Can you work these out from the model? Positions are in its coordinate system, mm. A direction names the side the tool comes from. Coordinates: 2 decimals unless noted, no trailing zeros. Order: outer loops, then holes, each group sorted by start corner. A loop starts at its lowest first (then second) coordinate and runs counter-clockwise, first axis right, second up. Notation, with made-up numbers: (33.25, 73) -> (86.25, 73) arc R20 cw to (86.25, 106) -> close; hole circle Ø9 at (22.25, 46). An arc over 180 degrees is marked (long way). Use a Markdown table: item, result. Add a question column.
1. Suppose I cut it at C-C, the plane z = 7. List the corners of the cut face in (x, y) for me.
2. Suppose I cut it at B-B, the plane y = 62.5. List the corners of the cut face in (x, z) for me, then the cut area to 3 significant figures.
3. If I drill on line 1 along Y through (x, z) = (0, -8); line 2 along X through (y, z) = (-31.25, -0.2); line 3 along Z through (x, y) = (33, 12.5), over which ranges is the centre line in solid material (lowest first)? Write a range as from..to.
4. For faces 4 (the flat face through (-17, -46, 1)), 5 (the flat face through (-45, -16, -9)), 6 (the cylindrical face through (-11.923, 53.692, -6.535)), which set-ups out of +Z, -Z, +X, -X, +Y, -Y let a thin tool reach every point of the face, with its end or its side?
5. We'd pull the mould along X, two halves only. Please class faces 1 (the cylindrical face through (-28, -21, 7)), 2 (the flat face through (-37, -41, -4)), 3 (the conical face through (-9, 40, 8)): pulls with the +X half, pulls with the -X half, needs draft (parallel to the pull), parting line crosses it, or undercut.
6. For pin 1 Ø11.5 at (x, y) = (54.13, -31.25) entering from +Z; pin 2 Ø8 at (x, z) = (-9, -7) entering from -Y; pin 3 Ø6 at (x, z) = (42, -2) entering from -Y; pin 4 Ø6 at (x, y) = (-20, 38) entering from +Z, each with a flat end and sliding along its axis, tell me the tip position at first contact or that it passes through.
Autodesk Inventor part; units mm, degrees
ref_plane "YZ Plane" through (0, 0, 0) normal (1, 0, 0) x (0, 1, 0)
ref_plane "XZ Plane" through (0, 0, 0) normal (0, 1, 0) x (-1, 0, 0)
ref_plane "XY Plane" through (0, 0, 0) normal (0, 0, 1) x (1, 0, 0)
sketch "Sketch1" plane through (-195.9052, -159.4976, -9) normal (0, 0, 1) x (1, 0, 0)
  circle A0 centre (195.9052, 159.4976) radius 70
  dimension "d29" = 140
extrude "ExtrusionBlind1" add sketch "Sketch1" along normal blind 18
sketch "Sketch2" plane through (-195.9052, -159.4976, -9) normal (0, 0, 1) x (1, 0, 0)
  circle A0 centre (195.9052, 159.4976) radius 55
  circle A1 centre (195.9052, 159.4976) radius 83.1126
  circle A2 centre (195.9052, 159.4976) radius 70
  dimension "d30" = 166.2252
  dimension "d31" = 110
extrude "ExtrusionBlind2" cut sketch "Sketch2" along normal blind 5 contours A1 | A2
sketch "Sketch3" plane through (-195.9052, -159.4976, -9) normal (0, 0, 1) x (1, 0, 0)
  circle A0 centre (195.9052, 159.4976) radius 30
  circle A1 centre (195.9052, 159.4976) radius 55
  dimension "d32" = 60
extrude "ExtrusionThru1" cut sketch "Sketch3" along normal through all contours A0
sketch "Sketch4" plane through (-195.9052, -159.4976, -9) normal (0, 0, 1) x (1, 0, 0)
  circle A0 centre (195.9052, 159.4976) radius 37.5
  circle A1 centre (195.9052, 159.4976) radius 55
  dimension "d33" = 75
extrude "ExtrusionBlind3" cut sketch "Sketch4" along normal blind 11 contours A0
sketch "Sketch5" plane through (-195.9052, -159.4976, -9) normal (0, 0, 1) x (1, 0, 0)
  circle A0 centre (195.9052, 159.4976) radius 47.5
  circle A1 centre (195.9052, 159.4976) radius 55
  dimension "d34" = 95
extrude "ExtrusionBlind4" cut sketch "Sketch5" along normal blind 3 contours A0
sketch "Sketch6" plane through (0, 0, -4) normal (0, 0, -1) x (-1, 0, 0)
  point P0 (0, -62.5)
hole "Hole1" at (0, -62.5, -4) direction (0, 0, 1) diameter 9 end through all
pattern_circular "PolarArray1" count 6 over 360 about axis through (0, 0, -9) along (0, 0, -1) of "Hole1"
sketch "Sketch9" plane through (0, 0, 9) normal (0, 0, 1) x (1, 0, 0)
  circle A0 centre (0, 0) radius 35
  circle A1 centre (0, 0) radius 47.5
  dimension "d35" = 70
extrude "ExtrusionBlind5" cut sketch "Sketch9" against normal blind 5 contours A0
sketch "Sketch10" plane through (0, 0, 9) normal (0, 0, 1) x (1, 0, 0)
  circle A0 centre (0, 0) radius 48
  circle A1 centre (0, 0) radius 87.5498
  circle A2 centre (0, 0) radius 55
  dimension "d36" = 175.0996
  dimension "d37" = 96
extrude "ExtrusionBlind6" cut sketch "Sketch10" against normal blind 8 contours A1 | A2
chamfer "Chamfer1" distance 8 angle 45 1 edges at (-48, 0, 9)
properties part number "7055-192 PART1" material "Steel, Mild"
Worked out:
| question | item | result |
|---|---|---|
| 1 | outline | circle Ø84 at (0, 0); hole circle Ø70 at (0, 0) |
| 2 | outline | (-31.52, -4) -> (-4.5, -4) -> (-4.5, 1) -> (-31.52, 1) -> close; (4.5, -4) -> (31.52, -4) -> (31.52, 1) -> (4.5, 1) -> close |
| 2 | area | 270 mm² |
| 3 | line 1 | y = -55..-47.5, 47.5..55 |
| 3 | line 2 | x = -62.64..-58.63, -49.63..-20.73, 20.73..49.63, 58.63..62.64 |
| 3 | line 3 | z = 2..9 |
| 4 | face 4 | +Z |
| 4 | face 5 | -Z, +X, -X, +Y, -Y |
| 4 | face 6 | -Z |
| 5 | face 1 | undercut |
| 5 | face 2 | needs draft |
| 5 | face 3 | parting line crosses it |
| 6 | pin 1 | stops at z = 1 |
| 6 | pin 2 | stops at y = -69.71 |
| 6 | pin 3 | stops at y = -58.13 |
| 6 | pin 4 | stops at z = 9 |
